For this review, take the finished solid that the model builds, in its own axes (mm). Face numbers are marked on the shaded views. A direction names the side the tool comes from. Coordinates: 2 decimals unless noted, no trailing zeros. Loops run counter-clockwise (first coordinate to the right, second up) from the corner with the lowest first, then second, coordinate; pieces in that order, holes last. Notation, with made-up numbers: (41.25, 36) - (86.25, 36) arc R28 ccw to (86.25, 57) - close; hole circle Ø6 at (64.25, 83). An arc over 180 degrees is marked (long way). One line per item, written item: value. Start each with the question number.
1. Take a section at B-B, the plane z = 12. State the section outline as (x, y) points, and give its area (3 significant figures).
2. Take a section at A-A, the plane y = 4.25. State the section outline as (x, z) points, and give its area (3 significant figures).
3. The part is to be moulded in two halves that separate along X. For the marked faces 4, 5, 6 and 7, say which applies: released by +X, released by -X, zero draft, split by the parting line, or undercut.
4. For the marked faces 1, 2 and 3, list the 3-axis set-ups (+Z, -Z, +X, -X, +Y, -Y) from which the entire face can be reached by the end or side of a thin tool; tool diameter is ignored.
5. Take a section at C-C, the plane x = -5. State the section outline as (y, z) points, and give its area (3 significant figures).
6. Insertion check: pin 1 (5 mm diameter, centred on y = -10.5, z = 24.5, fed in from +X); pin 2 (9.5 mm diameter, centred on x = 28.45, z = 39.02, fed in from -Y); pin 3 (5 mm diameter, centred on y = -1.5, z = 23.5, fed in from -X). Each pin has a flat end and moves straight along its axis. Give the tip position at first contact, or say it passes through.
7. To check wall thickness, follow line 1 (X direction, y = -6.5, z = 13); line 2 (Y direction, x = 1.5, z = 19); line 3 (X direction, y = 4, z = 27.5). State the ranges of each line that lie inside material, in increasing order. Write a range as from..to.
8. Take a section at D-D, the plane x = -18. State the section outline as (y, z) points.
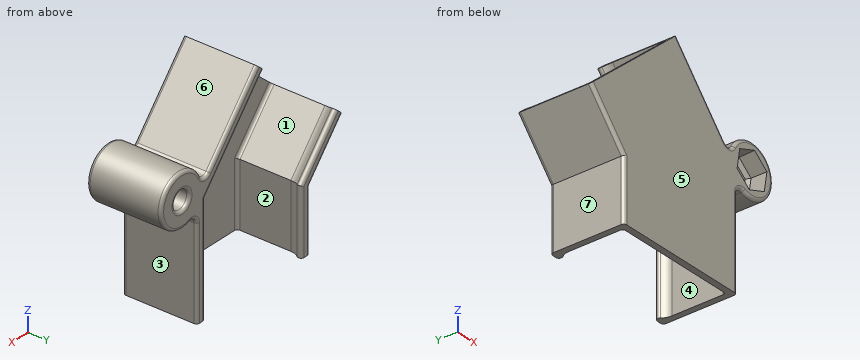
```python
from build123d import *
from OCP.BRepFilletAPI import BRepFilletAPI_MakeChamfer

# Parameters (mm, degrees)
SKETCH4_R           = 2.9999999999999982
BOSS_EXTRUDE2_DEPTH = 24
CUT_EXTRUDE2_DEPTH  = 6
CUT_EXTRUDE2_DRAFT  = -2.0000000000000044
CHAMFER1_SIZE       = 1
CHAMFER1_SIZE2      = 1.0368159552784713
FILLET8_R           = 1


with BuildPart() as part:
    # Sweep1: sweep along a path in Sketch3
    with BuildLine(Plane(origin=(0, 0, 0), x_dir=(1, 0, 0), z_dir=(0, 1, 0))) as sweep1_path:
        Line((0, 0), (3.43e-15, -28.397932341701697))
        Line((3.43e-15, -28.397932341701697), (-18.606512367640427, -49.85114326213761))
    # Sketch1 → Sweep1 (sweep)
    with BuildSketch(Plane.XY):
        with BuildLine():
            Line((-19.500000000000004, -12.023018516113881), (19.500000000000004, -12.023018516113881))
            ThreePointArc((19.500000000000004, -12.023018516113881), (20.207106781186553, -11.730125297300427), (20.499999999999996, -11.02301851611388))
            Line((20.499999999999996, -11.02301851611388), (20.5, 5.476981483886118))
            ThreePointArc((20.5, 5.476981483886118), (20.235010721400677, 6.998390104086923), (19.471251471279412, 8.34061784752248))
            ThreePointArc((19.471251471279412, 8.34061784752248), (19.338106653385996, 9.403382916597337), (20.242640687119284, 9.976981483886115))
            Line((20.242640687119284, 9.976981483886115), (21.5, 9.976981483886117))
            ThreePointArc((21.5, 9.976981483886117), (22.207106781186546, 9.684088265072665), (22.5, 8.976981483886117))
            Line((22.5, 8.976981483886117), (22.500000000000004, -13.023018516113874))
            ThreePointArc((22.500000000000004, -13.023018516113874), (22.20710678118655, -13.730125297300424), (21.5, -14.023018516113883))
            Line((21.5, -14.023018516113883), (-21.5, -14.023018516113883))
            ThreePointArc((-21.5, -14.023018516113883), (-22.20710678118655, -13.730125297300424), (-22.500000000000004, -13.023018516113874))
            Line((-22.500000000000004, -13.023018516113874), (-22.5, 8.976981483886117))
            ThreePointArc((-22.5, 8.976981483886117), (-22.207106781186546, 9.684088265072665), (-21.5, 9.976981483886117))
            Line((-21.5, 9.976981483886117), (-20.242640687119284, 9.976981483886115))
            ThreePointArc((-20.242640687119284, 9.976981483886115), (-19.338106653385996, 9.403382916597337), (-19.471251471279412, 8.34061784752248))
            ThreePointArc((-19.471251471279412, 8.34061784752248), (-20.235010721400677, 6.998390104086923), (-20.5, 5.476981483886118))
            Line((-20.5, 5.476981483886118), (-20.499999999999996, -11.02301851611388))
            ThreePointArc((-20.499999999999996, -11.02301851611388), (-20.207106781186553, -11.730125297300429), (-19.500000000000004, -12.023018516113881))
        make_face()
    sweep(path=sweep1_path.line, transition=Transition.RIGHT)

    # Sketch4 → Boss-Extrude2 (add, through all)
    with BuildSketch(Plane(origin=(0, -14.023018516113883, 0), x_dir=(-1, 0, 0), z_dir=(0, -1, 0))):
        with BuildLine():
            Line((-21.5, -34.67531871716202), (-21.5, -29.459053367546638))
            Line((-21.5, -29.459053367546638), (-22.500000000000004, -29.459053367546638))
            ThreePointArc((-22.500000000000004, -29.459053367546638), (-23.388194611615152, -31.12154811290928), (-25.26388877835841, -31.307423983602327))
            ThreePointArc((-25.263888778358414, -31.307423983602334), (-36.264928425658965, -41.93350635482782), (-20.991916583156645, -42.753023981442176))
            ThreePointArc((-20.991916583156645, -42.75302398144217), (-19.45313679656983, -41.66447668579883), (-17.692872887894488, -42.33845696613024))
            Line((-17.692872887894488, -42.33845696613024), (-16.93742313675424, -41.68325037771543))
            Line((-16.93742313675424, -41.68325037771543), (-21.5, -36.42262324599441))
            Line((-21.5, -36.42262324599441), (-21.5, -34.67531871716202))
        make_face()
        with Locations(Location((-28.449921846657176, -39.01662206592069, 0), (0, 0, 90))):
            Circle(SKETCH4_R, mode=Mode.SUBTRACT)
    extrude(amount=-BOSS_EXTRUDE2_DEPTH)


with BuildPart() as cut_extrude2_tool:
    # Sketch5 → Cut-Extrude2 (with draft: the straight prism first)
    with BuildSketch(Plane(origin=(0, -14.023018516113883, 0), x_dir=(-1, 0, 0), z_dir=(0, -1, 0))):
        Polygon((-29.501650461083923, -45.27978422691646), (-23.551728614426768, -43.05902684439915), (-22.500000000000025, -36.79586468340338), (-27.39819323223043, -32.75345990492492), (-33.348115078887595, -34.974217287442244), (-34.39984369331434, -41.237379448438006), align=None)
    extrude(amount=-CUT_EXTRUDE2_DEPTH)
    # Cut-Extrude2: the draft: its side faces are tilted about the plane it starts from
    cut_extrude2_sides = [cut_extrude2_tool.faces().sort_by_distance(p)[0] for p in [
        (26.526689538, -11.023018516, 44.169405536),
        (23.025864307, -11.023018516, 39.927445764),
        (24.949096616, -11.023018516, 34.774662294),
        (30.373154156, -11.023018516, 33.863838596),
        (33.873979386, -11.023018516, 38.105798368),
        (31.950747077, -11.023018516, 43.258581838),
    ]]
    draft(cut_extrude2_sides, Plane(origin=(0, -14.023018516113883, 0), x_dir=(-1, 0, 0), z_dir=(0, -1, 0)), CUT_EXTRUDE2_DRAFT)


with BuildPart() as part_1:
    add(part.part)

    # Cut-Extrude2: cut by cut_extrude2_tool
    add(cut_extrude2_tool.part, mode=Mode.SUBTRACT)

    # Chamfer1: one chamfer whose edges measure the first distance from different faces: ONE call of the kernel's chamfer builder (chamfer() names one face for all edges)
    chamfer1_edges_1 = [part_1.edges().sort_by_distance(p)[0] for p in [
        (33.667347826415636, -8.023018516113883, 38.14049654729082),
    ]]
    chamfer1_side_1 = [part_1.faces().sort_by_distance(p)[0] for p in [
        (33.77133231943445, -11.042436068122724, 38.123035165331785),
    ]]
    chamfer1_edges_2 = [part_1.edges().sort_by_distance(p)[0] for p in [
        (30.299887880499114, -8.023018516113883, 34.060135865770036),
    ]]
    chamfer1_side_2 = [part_1.faces().sort_by_distance(p)[0] for p in [
        (30.336758126646806, -11.042436068122724, 33.96135196223658),
    ]]
    chamfer1_edges_3 = [part_1.edges().sort_by_distance(p)[0] for p in [
        (25.08246190074066, -8.023018516113883, 34.936261384399906),
    ]]
    chamfer1_side_3 = [part_1.faces().sort_by_distance(p)[0] for p in [
        (25.015347653869544, -11.042436068122724, 34.854938862825485),
    ]]
    chamfer1_edges_4 = [part_1.edges().sort_by_distance(p)[0] for p in [
        (23.232495866898734, -8.023018516113883, 39.89274758455057),
    ]]
    chamfer1_side_4 = [part_1.faces().sort_by_distance(p)[0] for p in [
        (23.12851137387992, -11.042436068122724, 39.91020896650961),
    ]]
    chamfer1_edges_5 = [part_1.edges().sort_by_distance(p)[0] for p in [
        (26.599955812815256, -8.023018516113883, 43.97310826607136),
    ]]
    chamfer1_side_5 = [part_1.faces().sort_by_distance(p)[0] for p in [
        (26.56308556666756, -11.042436068122724, 44.07189216960481),
    ]]
    chamfer1_edges_6 = [part_1.edges().sort_by_distance(p)[0] for p in [
        (31.81738179257371, -8.023018516113883, 43.09698274744148),
    ]]
    chamfer1_side_6 = [part_1.faces().sort_by_distance(p)[0] for p in [
        (31.88449603944482, -11.042436068122724, 43.178305269015894),
    ]]
    chamfer1 = BRepFilletAPI_MakeChamfer(part_1.part.solid().wrapped)
    for e in chamfer1_edges_1:
        chamfer1.Add(CHAMFER1_SIZE, CHAMFER1_SIZE2, e.wrapped, chamfer1_side_1[0].wrapped)  # the first distance lies on this face
    for e in chamfer1_edges_2:
        chamfer1.Add(CHAMFER1_SIZE, CHAMFER1_SIZE2, e.wrapped, chamfer1_side_2[0].wrapped)  # the first distance lies on this face
    for e in chamfer1_edges_3:
        chamfer1.Add(CHAMFER1_SIZE, CHAMFER1_SIZE2, e.wrapped, chamfer1_side_3[0].wrapped)  # the first distance lies on this face
    for e in chamfer1_edges_4:
        chamfer1.Add(CHAMFER1_SIZE, CHAMFER1_SIZE2, e.wrapped, chamfer1_side_4[0].wrapped)  # the first distance lies on this face
    for e in chamfer1_edges_5:
        chamfer1.Add(CHAMFER1_SIZE, CHAMFER1_SIZE2, e.wrapped, chamfer1_side_5[0].wrapped)  # the first distance lies on this face
    for e in chamfer1_edges_6:
        chamfer1.Add(CHAMFER1_SIZE, CHAMFER1_SIZE2, e.wrapped, chamfer1_side_6[0].wrapped)  # the first distance lies on this face
    add(Compound.cast(chamfer1.Shape()), mode=Mode.REPLACE)

    # Fillet8
    # the kernel refuses this fillet: 1 mm, written as the material it takes off along each edge
    with BuildSketch(Plane(origin=(24.500000000000004, -14.023018516113883, 29.459053367546634), x_dir=(-0.31457819430358575, 0, -0.9492315627225506), z_dir=(0.9492315627225506, 0, -0.31457819430358575))) as fillet8_piece_1:
        with BuildLine():
            CenterArc((2 + FILLET8_R, FILLET8_R), FILLET8_R, 180, 90)
            Line((2, FILLET8_R), (2, 0))
            Line((2, 0), (2 + FILLET8_R, 0))
        make_face()
    revolve(axis=Axis((24.500000000000004, -14.023018516113883, 29.459053367546634), (0, 1, 0)), revolution_arc=184.1188230563678, mode=Mode.SUBTRACT)
    with BuildSketch(Plane(origin=(24.500000000000004, 9.976981483886117, 29.459053367546634), x_dir=(-0.31457819430358197, 0, -0.9492315627225518), z_dir=(0.9492315627225518, 0, -0.31457819430358197))) as fillet8_piece_2:
        with BuildLine():
            CenterArc((2.000000000000001 + FILLET8_R, -FILLET8_R), FILLET8_R, 90, 90)
            Line((2.000000000000001 + FILLET8_R, 3.55e-15), (2.000000000000001, 3.55e-15))
            Line((2.000000000000001, 3.55e-15), (2.000000000000001, -FILLET8_R))
        make_face()
    revolve(axis=Axis((24.500000000000004, 9.976981483886117, 29.459053367546634), (0, 1, 0)), revolution_arc=184.11882305636792, mode=Mode.SUBTRACT)
    with BuildSketch(Plane(origin=(19.20377239017497, -14.023018516113883, 43.64887014295982), x_dir=(0.8940720964908377, 0, -0.4479230807588265), z_dir=(0.4479230807588265, 0, 0.8940720964908377))) as fillet8_piece_3:
        with BuildLine():
            CenterArc((2.0000000000000004 + FILLET8_R, FILLET8_R), FILLET8_R, 180, 90)
            Line((2.000000000000001, FILLET8_R), (2.0000000000000004, 0))
            Line((2.0000000000000004, 0), (2.0000000000000004 + FILLET8_R, 0))
        make_face()
    revolve(axis=Axis((19.20377239017497, -14.023018516113883, 43.64887014295982), (0, 1, 0)), revolution_arc=184.1188230563678, mode=Mode.SUBTRACT)
    with BuildSketch(Plane(origin=(19.20377239017497, 9.976981483886117, 43.64887014295982), x_dir=(0.8940720964908377, 0, -0.4479230807588265), z_dir=(0.4479230807588265, 0, 0.8940720964908377))) as fillet8_piece_4:
        with BuildLine():
            CenterArc((2.0000000000000004 + FILLET8_R, -FILLET8_R), FILLET8_R, 90.00000000000018, 89.99999999999983)
            Line((2.0000000000000004 + FILLET8_R, 0), (2.0000000000000004, 0))
            Line((2.0000000000000004, 0), (2.000000000000001, -FILLET8_R))
        make_face()
    revolve(axis=Axis((19.20377239017497, 9.976981483886117, 43.64887014295982), (0, 1, 0)), revolution_arc=184.1188230563678, mode=Mode.SUBTRACT)
    with BuildSketch(Plane(origin=(28.449921846657183, -14.023018516113883, 39.0166220659207), x_dir=(-0.3819443891792063, 0, -0.9241853080278452), z_dir=(-0.9241853080278452, 0, 0.3819443891792063))) as fillet8_piece_5:
        with BuildLine():
            CenterArc((8.341615058531193 - FILLET8_R, -FILLET8_R), FILLET8_R, 0, 90)
            Line((8.34161505853119, -FILLET8_R), (8.341615058531193, 0))
            Line((8.341615058531193, 0), (8.341615058531193 - FILLET8_R, 0))
        make_face()
    revolve(axis=Axis((28.449921846657183, -14.023018516113883, 39.0166220659207), (0, -1, 0)), revolution_arc=265.84366585936306, mode=Mode.SUBTRACT)
    with BuildSketch(Plane(origin=(28.449921846657183, 9.976981483886117, 39.0166220659207), x_dir=(-0.3819443891792063, 0, -0.9241853080278452), z_dir=(-0.9241853080278452, 0, 0.3819443891792063))) as fillet8_piece_6:
        with BuildLine():
            CenterArc((8.341615058531193 - FILLET8_R, FILLET8_R), FILLET8_R, 270.00000000000034, 89.99999999999966)
            Line((8.341615058531193 - FILLET8_R, 0), (8.341615058531193, 0))
            Line((8.341615058531193, 0), (8.34161505853119, FILLET8_R))
        make_face()
    revolve(axis=Axis((28.449921846657183, 9.976981483886117, 39.0166220659207), (0, -1, 0)), revolution_arc=265.84366585936306, mode=Mode.SUBTRACT)
    with BuildSketch(Plane(origin=(28.449921846657176, 9.976981483886117, 39.01662206592069), x_dir=(0, 0, -1), z_dir=(-1, 0, 0))) as fillet8_piece_7:
        with BuildLine():
            CenterArc((3 + FILLET8_R, FILLET8_R), FILLET8_R, 180, 90)
            Line((3 + FILLET8_R, 0), (3, 0))
            Line((3, 0), (3, FILLET8_R))
        make_face()
    revolve(axis=Axis((28.449921846657176, 9.976981483886117, 39.01662206592069), (0, -1, 0)), mode=Mode.SUBTRACT)


solid = part_1.part
```
Solutions:
1. outline: (-22.5, -13.02) arc R1 ccw to (-21.5, -14.02) - (21.5, -14.02) arc R1 ccw to (22.5, -13.02) - (22.5, 8.98) arc R1 ccw to (21.5, 9.98) - (20.24, 9.98) arc R1 ccw to (19.47, 8.34) arc R4.5 cw to (20.5, 5.48) - (20.5, -11.02) arc R1 cw to (19.5, -12.02) - (-19.5, -12.02) arc R1 cw to (-20.5, -11.02) - (-20.5, 5.48) arc R4.5 cw to (-19.47, 8.34) arc R1 ccw to (-20.24, 9.98) - (-21.5, 9.98) arc R1 ccw to (-22.5, 8.98) - close
1. area: 183 mm2
2. outline: (-35.6, 35.11) - (-22.5, 20) - (-22.5, 0) - (-20.5, 0) - (-20.5, 20.75) - (-34.09, 36.42) - close; (-3.12, 63.28) - (20.5, 36.05) - (20.5, 0) - (22.5, 0) - (22.5, 29.46) arc R2 cw to (25.26, 31.31) arc R8.34 ccw (long way) to (20.99, 42.75) arc R2 cw to (17.69, 42.34) - (-1.61, 64.59) - close; hole circle Ø6 at (28.45, 39.02)
2. area: 415 mm2
3. face 4: undercut
3. face 5: zero draft
3. face 6: undercut
3. face 7: released by -X
4. face 1: +Z
4. face 2: +Z, -Z
4. face 3: -Z, +X, +Y, -Y
5. outline: (-14.02, 0) - (-12.02, 0) - (-12.02, 61.65) - (-14.02, 61.65) - close
5. area: 123 mm2
6. pin 1: x = 22.5
6. pin 2: y = -8.49
6. pin 3: x = -27.7
7. line 1: -22.5..-20.5, 20.5..22.5
7. line 2: -14.02..-12.02
7. line 3: -29..-26.36, 20.5..22.5
8. outline: (-14.02, 0) - (-12.02, 0) - (-12.02, 50.38) - (-14.02, 50.38) - close
